Can you work these out from the model? Positions are in its coordinate system, mm. A direction names the side the tool comes from. Give positions to 0.01 mm unless a question says otherwise; leave off trailing zeros. Order: outer loops, then holes, each group sorted by start corner. A loop starts at its lowest first (then second) coordinate and runs counter-clockwise, first axis right, second up. Notation, with made-up numbers: M 68,67.25 L 100,67.25 A31 ccw 100,102.25 Z; hole C 12,57.25 d1. An arc over 180 degrees is marked long. Answer as a JSON object with one key per item and string values.
Autodesk Inventor part; units mm, degrees
ref_plane "YZ Plane" through (0, 0, 0) normal (1, 0, 0) x (0, 1, 0)
ref_plane "XZ Plane" through (0, 0, 0) normal (0, 1, 0) x (-1, 0, 0)
ref_plane "XY Plane" through (0, 0, 0) normal (0, 0, 1) x (1, 0, 0)
sketch "Sketch1" plane through (0, 0, 0) normal (0, 0, 1) x (1, 0, 0)
  arc A0 (-39.1074, 3.3431) -> (-3.3431, 39.1074) centre (0, 0) ccw
  line L0 (0, 0) -> (30.017, 0) construction
  line L1 (-39.1074, 3.3431) -> (-3.3431, 39.1074)
  line L2 (0, 0) -> (39.25, 0) construction
  circle A1 centre (22.8042, -22.8042) radius 3
  circle A2 centre (-26.9378, -17.7318) radius 3
  circle A3 centre (17.7318, 26.9378) radius 3
  dimension "d0" = 78.5
  dimension "d6" = 6
  dimension "d9" = 6
  dimension "d10" = 6
extrude "Extrusion1" add sketch "Sketch1" along normal blind 10
sketch "Sketch2" plane through (0, 0, 10) normal (0, 0, 1) x (1, 0, 0)
  circle A0 centre (17.7318, 26.9378) radius 3
  circle A1 centre (17.7318, 26.9378) radius 5
  circle A2 centre (22.8042, -22.8042) radius 3
  circle A3 centre (22.8042, -22.8042) radius 5
  circle A4 centre (-26.9378, -17.7318) radius 3
  circle A5 centre (-26.9378, -17.7318) radius 5
  point P0 (0, 0)
  dimension "d13" = 10
  dimension "d14" = 10
  dimension "d15" = 10
extrude "Extrusion2" cut sketch "Sketch2" against normal blind 5 contours A1
extrude "Extrusion3" cut sketch "Sketch2" against normal blind 5 contours A5
extrude "Extrusion4" cut sketch "Sketch2" against normal blind 5 contours A3
sketch "Sketch3" plane through (0, 0, 10) normal (0, 0, 1) x (1, 0, 0)
  line L0 (0, 0) -> (25, 0) construction
  circle A0 centre (-12.5, -21.6506) radius 2
  arc A1 (-39.1074, 3.3431) -> (-3.3431, 39.1074) centre (0, 0) ccw
  circle A2 centre (25, 0) radius 2
  circle A3 centre (-12.5, 21.6506) radius 2
  dimension "d24" = 4
  dimension "d27" = 360
extrude "Extrusion5" cut sketch "Sketch3" against normal through all contours A0
extrude "Extrusion6" cut sketch "Sketch3" against normal through all contours A2
extrude "Extrusion7" cut sketch "Sketch3" against normal through all contours A3
sketch "Sketch4" plane through (0, 0, 0) normal (0, 0, -1) x (-1, 0, 0)
  circle A0 centre (12.5, 21.6506) radius 2
  circle A1 centre (12.5, 21.6506) radius 4
  circle A2 centre (-25, 0) radius 2
  circle A3 centre (-25, 0) radius 4
  circle A4 centre (12.5, -21.6506) radius 2
  circle A5 centre (12.5, -21.6506) radius 4
  point P0 (0, 0)
  dimension "d35" = 8
  dimension "d36" = 8
  dimension "d37" = 8
extrude "Extrusion8" cut sketch "Sketch4" against normal blind 5 contours A1
extrude "Extrusion9" cut sketch "Sketch4" against normal blind 5 contours A5
extrude "Extrusion10" cut sketch "Sketch4" against normal blind 5 contours A3
sketch "Sketch5" plane through (0, 0, 10) normal (0, 0, 1) x (1, 0, 0)
  circle A0 centre (17.7318, 26.9378) radius 3
  circle A1 centre (22.8042, -22.8042) radius 3
  circle A2 centre (-26.9378, -17.7318) radius 5
  arc A3 (12.2473, -17.7267) -> (11.0285, -27.6521) centre (11.6379, -22.6894) ccw
  arc A4 (-39.1074, 3.3431) -> (-3.3431, 39.1074) centre (0, 0) ccw
  arc A5 (-30.0025, -6.3107) -> (-23.4023, -14.1962) centre (17.7318, 26.9378) ccw
  line L0 (-38.9658, -4.7151) -> (-34.7002, -4.204)
  line L1 (-24.2556, -21.9514) -> (-29.8381, -25.5)
  circle A6 centre (-26.9378, -17.7318) radius 5
  arc A7 (-30.0025, -6.3107) -> (-34.7002, -4.204) centre (-34.1053, -9.1685) ccw
  arc A8 (12.2473, -17.7267) -> (22.2969, -17.83) centre (17.7318, 26.9378) ccw
  arc A9 (11.0285, -27.6521) -> (23.3114, -27.7784) centre (17.7318, 26.9378) ccw
  circle A10 centre (22.8042, -22.8042) radius 5
  dimension "d46" = 10
extrude "Extrusion11" cut sketch "Sketch5" against normal blind 5 contours A2 L1 A4 L0 A7 A5
extrude "Extrusion12" cut sketch "Sketch5" against normal blind 5 contours A8 A10 A9 A3 | A10
sketch "Sketch6" plane through (0, 0, 5) normal (0, 0, 1) x (1, 0, 0)
  circle A0 centre (17.7318, 26.9378) radius 3
  circle A1 centre (22.8042, -22.8042) radius 3
  circle A2 centre (-26.9378, -17.7318) radius 3
  arc A3 (12.0035, -19.7118) -> (22.4998, -19.8197) centre (17.7318, 26.9378) ccw
  arc A4 (11.2723, -25.6671) -> (23.1085, -25.7887) centre (17.7318, 26.9378) ccw
  arc A5 (12.2473, -17.7267) -> (11.0285, -27.6521) centre (11.6379, -22.6894) ccw
  arc A6 (12.0035, -19.7118) -> (11.2723, -25.6671) centre (11.6379, -22.6894) ccw
  arc A7 (-31.6436, -7.4538) -> (-24.8165, -15.6104) centre (17.7318, 26.9378) ccw
  arc A8 (-36.567, -10.8831) -> (-29.0592, -19.8531) centre (17.7318, 26.9378) ccw
  arc A9 (-30.0025, -6.3107) -> (-34.7002, -4.204) centre (-34.1053, -9.1685) ccw
  arc A10 (-31.6436, -7.4538) -> (-36.567, -10.8831) centre (-34.1053, -9.1685) ccw
  point P0 (0, 0)
  dimension "d69" = 106
  dimension "d70" = 6
  dimension "d71" = 6
extrude "Extrusion13" cut sketch "Sketch6" against normal blind 5 contours A1 A4 A6 A3
extrude "Extrusion14" cut sketch "Sketch6" against normal blind 5 contours A2 | A2 A8 A10 A7
sketch "Sketch7" plane through (0, 0, 10) normal (0, 0, 1) x (1, 0, 0)
  line L0 (-3.3431, 39.1074) -> (-39.1074, 3.3431)
  arc A0 (-29.8381, -25.5) -> (-3.3431, 39.1074) centre (0, 0) ccw
  line L1 (-2.5781, 39.1652) -> (-39.1652, 2.5781)
  line L2 (-2.5781, 39.1652) -> (49.1639, 39.1652) construction
  arc A1 (-39.1074, 3.3431) -> (-38.9658, -4.7151) centre (0, 0) ccw
  dimension "d77" = 135
extrude "Extrusion15" cut sketch "Sketch7" against normal blind 10
properties part number "Encoder Mount Base"
1) Thinking about a two-plate mould opening in X: for faces 4 (the face through (28.679, -26.797, 4.93)), 5 (the face through (-14.2, -23.4, 5)), 6 (the face through (-1, 1, 10)), which applies, pulls with the +X half, pulls with the -X half, needs draft (parallel to the pull), parting line crosses it, or undercut?
Results found:
{"face 4": "parting line crosses it", "face 5": "undercut", "face 6": "needs draft"}
2) I want a section at C-C on x = -13. Write out the boundary of the cut face in (y, z), and give its area (3 significant figures).
Results found:
{"outline": "M -37.03,0 L -25.62,0 L -25.62,5 L -23.59,5 L -23.59,10 L -37.03,10 Z; M -19.71,5 L -17.68,5 L -17.68,0 L 17.68,0 L 17.68,5 L 19.71,5 L 19.71,10 L -19.71,10 Z; M 23.59,5 L 25.62,5 L 25.62,0 L 28.74,0 L 28.74,10 L 23.59,10 Z", "area": "540 mm²"}
3) I want a section at A-A on y = 0. Write out the boundary of the cut face in (x, z), and give its area (3 significant figures).
Results found:
{"outline": "M -39.25,0 L 21,0 L 21,5 L 23,5 L 23,10 L -39.25,10 Z; M 27,5 L 29,5 L 29,0 L 39.25,0 L 39.25,10 L 27,10 Z", "area": "725 mm²"}
4) For faces 1 (the face through (-11.633, 17.746, 2.465)), 2 (the face through (25.78, -22.43, 2.46)), 3 (the face through (27.79, -22.41, 7.54)), which set-ups out of +Z, -Z, +X, -X, +Y, -Y let a thin tool reach every point of the face, with its end or its side?
Results found:
{"face 1": "-Z", "face 2": "+Z, -Z", "face 3": "+Z"}
5) I'm going to push flat-ended pins straight in: pin 1 Ø1.5 at (x, z) = (6.5, 3.5) entering from -Y; pin 2 Ø7 at (x, y) = (-12.5, 21.65) entering from -Z; pin 3 Ø2 at (y, z) = (-16.5, 4) entering from +X. Where does each tip first touch, or does it pass through?
Results found:
{"pin 1": "stops at y = -38.83", "pin 2": "stops at z = 5", "pin 3": "stops at x = 36.06"}
6) I need wall thicknesses on L1, parallel to Y at x = -13, z = 2.5; L2, parallel to Y at x = -12.5, z = 3.9; L3, parallel to X at y = 26, z = 6.75. Which ranges of each line are inside material? Lowest first, please.
Results found:
{"L1": "y = -37.03 to -25.62, -17.68 to 17.68, 25.62 to 28.74", "L2": "y = -37.21 to -25.65, -17.65 to 17.65, 25.65 to 29.24", "L3": "x = -15.74 to 12.82, 22.64 to 29.4"}
7) I want a section at B-B on z = 2.75. Write out the boundary of the cut face in (x, y), and give its area (3 significant figures).
Results found:
{"outline": "M -39.17,2.58 A39.25 ccw long -2.58,39.17 Z; hole M -36.57,-10.88 A66.18 ccw -29.06,-19.85 A3 ccw -24.82,-15.61 A60.17 cw -31.64,-7.45 A3 ccw Z; hole C -12.5,-21.65 d8; hole C -12.5,21.65 d8; hole M 11.27,-25.67 A52.99 ccw 23.11,-25.79 A3 ccw 22.5,-19.82 A47 cw 12,-19.71 A3 ccw Z; hole C 17.73,26.94 d6; hole C 25,0 d8", "area": "4,120 mm²"}
8) I want a section at D-D on y = -29. Write out the boundary of the cut face in (x, z), and give its area (3 significant figures).
Results found:
{"outline": "M -26.45,0 L 26.45,0 L 26.45,10 L -26.45,10 Z", "area": "529 mm²"}
